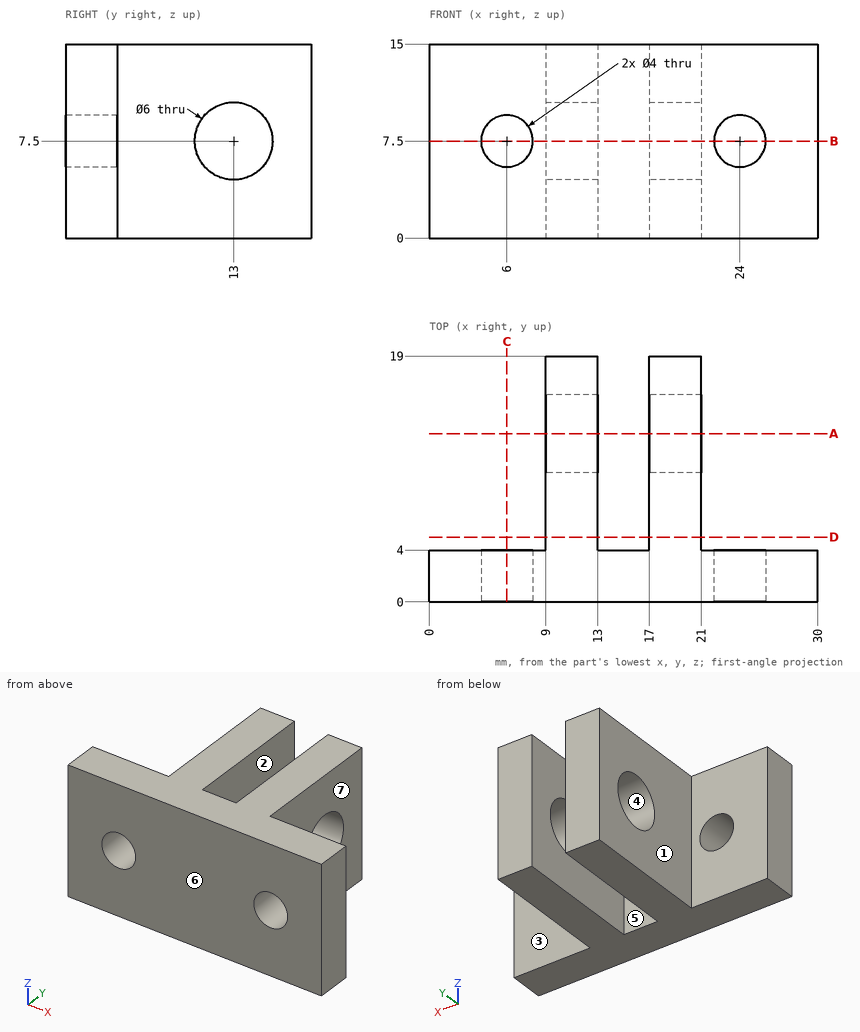
The figure shows three views and two pictorial views of one solid part (mm, origin at its lowest corner). Answer the questions. A direction names the side the tool comes from. Coordinates: 2 decimals unless noted, no trailing zeros. Order: outer loops, then holes, each group sorted by start corner. A loop starts at its lowest first (then second) coordinate and runs counter-clockwise, first axis right, second up.
Q1. A cutting plane is placed at B-B, the plane z = 7.5. Write down the section's boundary in (x, y).
Q2. For a pull along Y with two mould halves and no side action, classify the marked faces 4, 5, 6 and 7 as pulls with the +Y half, pulls with the -Y half, needs draft (parallel to the pull), parting line crosses it, or undercut.
Q3. Which of the six approach directions +Z, -Z, +X, -X, +Y, -Y give full straight-line access (tool end or side, diameter ignored) to the marked faces 1, 2 and 3?
Q4. A cutting plane is placed at C-C, the plane x = 6. Write down the section's boundary in (y, z).
Q5. Given P1, Ø3, axis at x = 25.5, z = 13, coming from the +Y side; P2, Ø4.5, axis at y = 8.5, z = 8, coming from the -X side; P3, Ø6, axis at x = 23.5, z = 3, coming from the -Y side, each flat-ended and moving along its own axis, determine where each tip first touches the part or whether it passes through.
Q6. A cutting plane is placed at D-D, the plane y = 5. Write down the section's boundary in (x, z).
Q7. A cutting plane is placed at A-A, the plane y = 13. Write down the section's boundary in (x, z).
Q8. Consider line 1 (X direction, y = 3, z = 7.5); line 2 (X direction, y = 14.25, z = 2.75); line 3 (Y direction, x = 10.2, z = 7.5). Determine where each line is inside the solid, lowest interval first.
Answers follow:
1. outline: (0, 0) - (4, 0) - (4, 4) - (0, 4) - close; (8, 0) - (22, 0) - (22, 4) - (21, 4) - (21, 10) - (17, 10) - (17, 4) - (13, 4) - (13, 10) - (9, 10) - (9, 4) - (8, 4) - close; (9, 16) - (13, 16) - (13, 19) - (9, 19) - close; (17, 16) - (21, 16) - (21, 19) - (17, 19) - close; (26, 0) - (30, 0) - (30, 4) - (26, 4) - close
2. face 4: undercut
2. face 5: pulls with the +Y half
2. face 6: pulls with the -Y half
2. face 7: needs draft
3. face 1: +Z, -Z, -X, +Y
3. face 2: +Z, -Z, +Y
3. face 3: +Z, -Z, +X, +Y
4. outline: (0, 0) - (4, 0) - (4, 5.5) - (0, 5.5) - close; (0, 9.5) - (4, 9.5) - (4, 15) - (0, 15) - close
5. P1: stops at y = 4
5. P2: stops at x = 9
5. P3: stops at y = 0
6. outline: (9, 0) - (13, 0) - (13, 15) - (9, 15) - close; (17, 0) - (21, 0) - (21, 15) - (17, 15) - close
7. outline: (9, 0) - (13, 0) - (13, 4.5) - (9, 4.5) - close; (9, 10.5) - (13, 10.5) - (13, 15) - (9, 15) - close; (17, 0) - (21, 0) - (21, 4.5) - (17, 4.5) - close; (17, 10.5) - (21, 10.5) - (21, 15) - (17, 15) - close
8. line 1: x = 0 to 4, 8 to 22, 26 to 30
8. line 2: x = 9 to 13, 17 to 21
8. line 3: y = 0 to 10, 16 to 19
